Part model, mm, in its own coordinate system. Face numbers are marked on the shaded views. Round coordinates to 2 decimals unless told otherwise and drop trailing zeros. Order: outer loops, then holes, each group sorted by start corner. A loop starts at its lowest first (then second) coordinate and runs counter-clockwise, first axis right, second up. Notation, with made-up numbers: (21.25, 42) - (28.25, 42) arc R16 cw to (28.25, 47) - close; hole circle Ø2 at (48, 32). An arc over 180 degrees is marked (long way). Return JSON: item names as keys, results as strings. Group by question number.
Item 1: Saw through at A-A on y = 31.5. List the corners of the cut face in (x, z).
Item 2: Saw through at D-D on z = -24.5. List the corners of the cut face in (x, y) (3 decimals), and give its area (3 significant figures).
Item 3: Saw through at C-C on y = -21.5. List the corners of the cut face in (x, z), and give its area (3 significant figures).
Item 4: Drop flat-ended pins along their axis: pin 1 (12 mm diameter, centred on x = 15, y = -37, fed in from -Z); pin 2 (2.5 mm diameter, centred on y = 27.5, z = -33.5, fed in from +X); pin 3 (10 mm diameter, centred on y = -11.5, z = 24.5, fed in from +X); pin 4 (12 mm diameter, centred on x = -21.5, z = -0.5, fed in from +Y). Give the stop position or say it passes through.
Item 5: Two-plate mould, pull along Y, no slides. Class the marked faces 1, 2, 3 and 4: released by +Y, released by -Y, zero draft, split by the parting line, or undercut.
Item 6: Saw through at B-B on z = 3.5. List the corners of the cut face in (x, y).
Item 7: Probe probe 1 along Y at (x, z) = (-6, 43.5); probe 2 along Z at (x, y) = (0, 58.15); probe 3 along X at (y, z) = (-11, 5). List the from-to ranges inside material, lowest first.
```python
from build123d import *

# Parameters (mm, degrees)
SKETCH_2_R               = 35
SKETCH_2_R_2             = 30
EXTRUDE_1_DEPTH          = 50
SKETCH_3_R               = 45
SKETCH_3_R_2             = 30
EXTRUDE_2_DEPTH          = 2
CUT_EXTRUDE_1_REACH      = 134.454
SKETCH_4_R               = 1.4
CUT_EXTRUDE_2_DEPTH      = 93.736184955
CUT_EXTRUDE_2_DEPTH_BACK = 93.736184955


with BuildPart() as part:
    # 草图1 → 旋转1 (revolve)
    with BuildSketch(Plane.XY, mode=Mode.PRIVATE) as revolve_1_sk:
        Polygon((-45, 0), (-30, 0), (-30, 60), (-50, 60), (-50, 55), (-35, 55), (-35, 3), (-45, 3), align=None)
    revolve(revolve_1_sk.sketch.rotate(Axis((0, -563.187180309, 0), (0, 1, 0)), 180), axis=Axis((0, -563.187180309, 0), (0, 1, 0)))

    # 草图2 → 凸台-拉伸1 (add)
    with BuildSketch(Plane.XZ):
        Circle(SKETCH_2_R)
        Circle(SKETCH_2_R_2, mode=Mode.SUBTRACT)
    extrude(amount=EXTRUDE_1_DEPTH)

    # 草图3 → 凸台-拉伸2 (add)
    with BuildSketch(Plane.XZ.offset(50)):
        Circle(SKETCH_3_R)
        Circle(SKETCH_3_R_2, mode=Mode.SUBTRACT)
    extrude(amount=EXTRUDE_2_DEPTH)

    # 草图4 → 切除-拉伸1 (cut, up to next)
    with BuildSketch(Plane(origin=(0, 60, 0), x_dir=(1, 0, 0), z_dir=(0, 1, 0)), mode=Mode.PRIVATE) as cut_extrude_1_sk1:
        with Locations(Location((0, 40, 0), (0, 0, 180))):
            Circle(SKETCH_4_R)
    cut_extrude_1_tool1 = extrude(cut_extrude_1_sk1.sketch, amount=-CUT_EXTRUDE_1_REACH, mode=Mode.PRIVATE) & part.part
    # 草图4 → 切除-拉伸1 (cut, up to next)
    with BuildSketch(Plane(origin=(0, 60, 0), x_dir=(1, 0, 0), z_dir=(0, 1, 0)), mode=Mode.PRIVATE) as cut_extrude_1_sk2:
        with Locations(Location((40, 0, 0), (0, 0, 180))):
            Circle(SKETCH_4_R)
    cut_extrude_1_tool2 = extrude(cut_extrude_1_sk2.sketch, amount=-CUT_EXTRUDE_1_REACH, mode=Mode.PRIVATE) & part.part
    # 草图4 → 切除-拉伸1 (cut, up to next)
    with BuildSketch(Plane(origin=(0, 60, 0), x_dir=(1, 0, 0), z_dir=(0, 1, 0)), mode=Mode.PRIVATE) as cut_extrude_1_sk3:
        with Locations(Location((0, -40, 0), (0, 0, 180))):
            Circle(SKETCH_4_R)
    cut_extrude_1_tool3 = extrude(cut_extrude_1_sk3.sketch, amount=-CUT_EXTRUDE_1_REACH, mode=Mode.PRIVATE) & part.part
    # 草图4 → 切除-拉伸1 (cut, up to next)
    with BuildSketch(Plane(origin=(0, 60, 0), x_dir=(1, 0, 0), z_dir=(0, 1, 0)), mode=Mode.PRIVATE) as cut_extrude_1_sk4:
        with Locations(Location((-40, 0, 0), (0, 0, 180))):
            Circle(SKETCH_4_R)
    cut_extrude_1_tool4 = extrude(cut_extrude_1_sk4.sketch, amount=-CUT_EXTRUDE_1_REACH, mode=Mode.PRIVATE) & part.part
    add(cut_extrude_1_tool1.solids().sort_by_distance((0, 60, -40))[0], mode=Mode.SUBTRACT)
    add(cut_extrude_1_tool2.solids().sort_by_distance((40, 60, 0))[0], mode=Mode.SUBTRACT)
    add(cut_extrude_1_tool3.solids().sort_by_distance((0, 60, 40))[0], mode=Mode.SUBTRACT)
    add(cut_extrude_1_tool4.solids().sort_by_distance((-40, 60, 0))[0], mode=Mode.SUBTRACT)

    # 草图5 → 切除-拉伸2 (cut, two sides)
    with BuildSketch(Plane.XY) as cut_extrude_2_sk:
        with BuildLine():
            Line((5, 45), (5, 15))
            ThreePointArc((5, 15), (0, 10), (-5, 15))
            Line((-5, 15), (-5, 45))
            ThreePointArc((-5, 45), (0, 50), (5, 45))
        make_face()
    extrude(amount=CUT_EXTRUDE_2_DEPTH, mode=Mode.SUBTRACT)
    extrude(cut_extrude_2_sk.sketch, amount=-CUT_EXTRUDE_2_DEPTH_BACK, mode=Mode.SUBTRACT)


solid = part.part
```
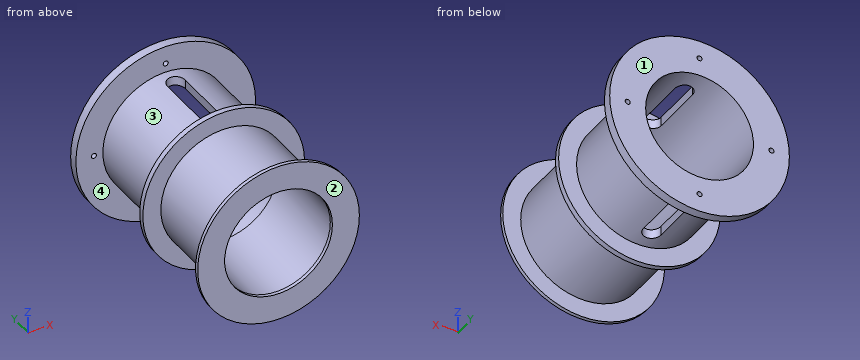
Filled in:
{
 "1": {"outline": "(-5, -34.64) - (-5, -29.58) arc R30 cw to (-5, 29.58) - (-5, 34.64) arc R35 ccw to start; (5, -34.64) arc R35 ccw to (5, 34.64) - (5, 29.58) arc R30 cw to (5, -29.58) - close"},
 "2": {"outline": "(-43.586, 55) - (-24.995, 55) - (-24.995, 3) - (-37.746, 3) - (-37.746, 0) - (-24.995, 0) - (-24.995, -50) - (-37.746, -50) - (-37.746, -52) - (-17.313, -52) - (-17.313, 60) - (-43.586, 60) - close; (17.313, -52) - (37.746, -52) - (37.746, -50) - (24.995, -50) - (24.995, 0) - (37.746, 0) - (37.746, 3) - (24.995, 3) - (24.995, 55) - (43.586, 55) - (43.586, 60) - (17.313, 60) - close", "area": "2,030 mm^2"},
 "3": {"outline": "circle Ø70 at (0, 0); hole circle Ø60 at (0, 0)", "area": "1,020 mm^2"},
 "4": {"pin 1": "stops at z = -33.82", "pin 2": "stops at x = 13.6", "pin 3": "stops at x = 29.06", "pin 4": "passes through"},
 "5": {"face 1": "released by +Y", "face 2": "released by -Y", "face 3": "undercut", "face 4": "undercut"},
 "6": {"outline": "(-49.88, 55) - (-34.82, 55) - (-34.82, 3) - (-44.86, 3) - (-44.86, 0) - (-34.82, 0) - (-34.82, -50) - (-44.86, -50) - (-44.86, -52) - (-29.8, -52) - (-29.8, 60) - (-49.88, 60) - close; (29.8, -52) - (44.86, -52) - (44.86, -50) - (34.82, -50) - (34.82, 0) - (44.86, 0) - (44.86, 3) - (34.82, 3) - (34.82, 55) - (49.88, 55) - (49.88, 60) - (29.8, 60) - close"},
 "7": {"probe 1": "y = -52 to -50, 0 to 3, 55 to 60", "probe 2": "z = -50 to -41.4, -38.6 to -30, 30 to 38.6, 41.4 to 50", "probe 3": "x = -34.64 to -29.58, 29.58 to 34.64"}
}
